```python
from build123d import *

# Parameters (mm, degrees)
F0_W     = 8
F0_H     = 8
F1_DEPTH = 125


with BuildPart() as f1:
    # F0 (on Front) → F1 (new body, symmetric)
    with BuildSketch(Plane.XZ):
        Polygon((-5, 17), (-5, 20), (-20, 20), (-20, 5), (-17, 5), (-17, 14.87868), (-17, 17), (-14.87868, 17), align=None)
        Polygon((-17, -5), (-20, -5), (-20, -20), (-5, -20), (-5, -17), (-14.87868, -17), (-17, -17), (-17, -14.87868), align=None)
        Polygon((20, -20), (20, -5), (17, -5), (17, -14.87868), (17, -17), (14.87868, -17), (5, -17), (5, -20), align=None)
        Polygon((20, 5), (20, 20), (5, 20), (5, 17), (14.87868, 17), (17, 17), (17, 14.87868), (17, 5), align=None)
        Polygon((17, 17), (14.87868, 17), (5.37868, 7.5), (7.5, 7.5), (7.5, 5.37868), (17, 14.87868), align=None)
        Polygon((-5.37868, 7.5), (-14.87868, 17), (-17, 17), (-17, 14.87868), (-7.5, 5.37868), (-7.5, 7.5), align=None)
        Polygon((-7.5, -5.37868), (-17, -14.87868), (-17, -17), (-14.87868, -17), (-5.37868, -7.5), (-7.5, -7.5), align=None)
        Polygon((17, -17), (17, -14.87868), (7.5, -5.37868), (7.5, -7.5), (5.37868, -7.5), (14.87868, -17), align=None)
        Polygon((7.5, 7.5), (5.37868, 7.5), (-5.37868, 7.5), (-7.5, 7.5), (-7.5, 5.37868), (-7.5, -5.37868), (-7.5, -7.5), (-5.37868, -7.5), (5.37868, -7.5), (7.5, -7.5), (7.5, -5.37868), (7.5, 5.37868), align=None)
        Rectangle(F0_W, F0_H, mode=Mode.SUBTRACT)
    extrude(amount=F1_DEPTH, both=True)


solid = f1.part
```
Model file for the job. Use its own axes, mm. A direction names the side the tool comes from. Round coordinates to 2 decimals unless told otherwise and drop trailing zeros. Loops run counter-clockwise (first coordinate to the right, second up) from the corner with the lowest first, then second, coordinate; pieces in that order, holes last. Notation, with made-up numbers: M -21,24.25 L 3,24.25 A11 cw 3,35.25 Z; hole C 60,58 d10. An arc over 180 degrees is marked long. Put each result on its own line as item: value. Start each with the question number.
Item 1: Cut at B-B (z = -12.5). List the corners of the cut face in (x, y).
Item 2: Drop flat-ended pins along their axis: P1, Ø5.5, axis at x = 0.5, y = -12, coming from the -Z side; P2, Ø2.5, axis at y = -26.5, z = -1.5, coming from the -X side. Give the stop position or say it passes through.
Item 3: Mould opens along Z. For faces 3 (the face through (-10.06, -1.75, 12.18)), 4 (the face through (12, -2, -20)), 5 (the face through (20, -2, 12)) say: released by +Z, released by -Z, zero draft, split by the parting line, or undercut.
Item 4: Cut at A-A (x = 1). List the corners of the cut face in (y, z).
Item 5: 3-axis set-ups, long thin cutter, end or side, ignore diameter. For faces 1 (the face through (0, -2, -4)), 2 (the face through (-12, -2, 20)): which of +Z, -Z, +X, -X, +Y, -Y reach the whole face in a straight line?
Item 6: Drill centre lines: line 1 along Z through (x, y) = (1, -62); line 2 along X through (y, z) = (51, -8); line 3 along X through (y, z) = (-70.5, -12). Where is each one in solid material? Low to high.
Answer block:
1. outline: M -20,-125 L -17,-125 L -17,125 L -20,125 Z; M -14.62,-125 L -10.38,-125 L -10.38,125 L -14.62,125 Z; M 10.38,-125 L 14.62,-125 L 14.62,125 L 10.38,125 Z; M 17,-125 L 20,-125 L 20,125 L 17,125 Z
2. P1: z = -7.5
2. P2: x = -7.5
3. face 3: undercut
3. face 4: released by -Z
3. face 5: zero draft
4. outline: M -125,-7.5 L 125,-7.5 L 125,-4 L -125,-4 Z; M -125,4 L 125,4 L 125,7.5 L -125,7.5 Z
5. face 1: +Y, -Y
5. face 2: +Z, +X, -X, +Y, -Y
6. line 1: -7.5 to -4, 4 to 7.5
6. line 2: -20 to -17, -10.12 to -5.88, 5.88 to 10.12, 17 to 20
6. line 3: -20 to -17, -14.12 to -9.88, 9.88 to 14.12, 17 to 20
